Geometry check sheet. Reference: the model listing, model coordinates, mm. A direction names the side the tool comes from. Coordinates: 2 decimals unless noted, no trailing zeros. Write each loop counter-clockwise with the first axis right and the second up, starting at its lowest first coordinate (ties: lowest second). Pieces come first, ordered by that corner, then holes. Notation, with made-up numbers: (-19.75, 4.5) -> (0.25, 4.5) arc R12 cw to (0.25, 27.5) -> close; hole circle Ø2 at (-20, -6.75). An arc over 180 degrees is marked (long way). One line per question, with ' | ' between items.
Autodesk Inventor part; units mm, degrees
ref_plane "YZ Plane" through (0, 0, 0) normal (1, 0, 0) x (0, 1, 0)
ref_plane "XZ Plane" through (0, 0, 0) normal (0, 1, 0) x (-1, 0, 0)
ref_plane "XY Plane" through (0, 0, 0) normal (0, 0, 1) x (1, 0, 0)
sketch "Sketch1" plane through (0, 0, 0) normal (1, 0, 0) x (0, 1, 0)
  line L0 (0, 0) -> (16, 0)
  line L1 (16, 0) -> (16, -52)
  line L2 (16, -52) -> (0, -52)
  line L3 (0, -10) -> (0, -10)
  line L4 (0, -10) -> (0, -25)
  line L5 (0, -25) -> (0, -25)
  line L6 (0, -42) -> (0, -42)
  line L7 (0, -42) -> (0, -27)
  line L8 (0, -27) -> (0, -27)
  line L9 (0, -10) -> (0, 0)
  line L10 (0, -52) -> (0, -42)
  line L11 (0, -27) -> (0, -25)
  dimension "d0" = 16
  dimension "d1" = 52
  dimension "d2" = 0
  dimension "d3" = 15
  dimension "d4" = 10
  dimension "d5" = 15
  dimension "d6" = 10
  dimension "d10" = 0
  dimension "d11" = 0
  dimension "d12" = 0
extrude "Extrusion1" add sketch "Sketch1" along normal blind 2
sketch "Sketch3" plane through (2, 0, 0) normal (1, 0, 0) x (0, 0, -1)
  circle A0 centre (10, 8) radius 2.5
  circle A1 centre (32, 8) radius 2.5
  circle A2 centre (44, 8) radius 2.5
  line L0 (0, 16) -> (0, 0)
  line L1 (52, 16) -> (0, 16)
  dimension "d18" = 5
  dimension "d19" = 5
  dimension "d20" = 5
  dimension "d21" = 10
  dimension "d22" = 8
  dimension "d23" = 8
  dimension "d24" = 22
  dimension "d25" = 8
  dimension "d26" = 12
extrude "Extrusion3" cut sketch "Sketch3" against normal blind 10
sketch "Sketch4" plane through (0, 0, 0) normal (-1, 0, 0) x (0, 0, 1)
  circle A0 centre (-63.5, 35) radius 2.5
  circle A1 centre (-77, 8) radius 1.5
  circle A2 centre (-65, 8) radius 1.5
  line L0 (-58, -1) -> (-58, 17)
  line L1 (-84, 17) -> (-58, 17)
  line L2 (-84, 17) -> (-84, -1)
  line L3 (-58, -1) -> (-84, -1)
  line L4 (-51.8335, 14.6577) -> (-40.3589, 16)
  line L5 (-52, 16) -> (0, 16)
  line L6 (-72.4772, 16.1758) -> (-72.4069, 41.1757)
  line L7 (-72.4069, 41.1757) -> (-56.407, 41.1307)
  line L8 (-56.407, 41.1307) -> (-56.4773, 16.1308)
  line L9 (-51.8335, 14.6577) -> (-72.4308, 32.6757)
  line L10 (-72.4069, 41.1757) -> (-56.407, 41.1307)
  line L11 (-56.407, 41.1307) -> (-56.4381, 30.0657)
  line L12 (-40.3589, 16) -> (-56.4381, 30.0657)
  point P0 (0, 0)
extrude "Extrusion4" add sketch "Sketch4" against normal blind 2 contours L6 L7 L8 L9 | L8 L12 L4 L9
properties part number "Mounting_wall"
1. Cross-section at B-B on x = 1.35. Record the boundary of the cut face in (y, z), and give its area (3 significant figures).
Worked answers:
outline: (0, -52) -> (14.8, -52) -> (32.68, -72.43) -> (41.18, -72.41) -> (41.13, -56.41) -> (30.07, -56.44) -> (16, -40.36) -> (16, 0) -> (0, 0) -> close; hole circle Ø5 at (8, -44); hole circle Ø5 at (8, -32); hole circle Ø5 at (8, -10); hole circle Ø5 at (35, -63.5) | area: 1,110 mm²
2. Cross-section at A-A on z = -32. Record the boundary of the cut face in (x, y).
Worked answers:
outline: (0, 0) -> (2, 0) -> (2, 5.5) -> (0, 5.5) -> close; (0, 10.5) -> (2, 10.5) -> (2, 16) -> (0, 16) -> close
3. Go/stop test with flat-tipped pins: P1, Ø1, axis at y = 17.5, z = -32, coming from the -X side; P2, Ø1, axis at x = 0.5, y = 14, coming from the -Z side. Record where each tip stops, or that it passes through.
Worked answers:
P1: through | P2: z = -52
4. Material ranges on line 1 (Y direction, x = 0.6, z = -10); line 2 (Z direction, x = 0.3, y = 8.5); line 3 (Z direction, x = 0.4, y = 9), recorded low to high. Write a range as from..to.
Worked answers:
line 1: 0..5.5, 10.5..16 | line 2: -52..-46.45, -41.55..-34.45, -29.55..-12.45, -7.55..0 | line 3: -52..-46.29, -41.71..-34.29, -29.71..-12.29, -7.71..0
5. Cross-section at D-D on z = -44. Record the boundary of the cut face in (x, y).
Worked answers:
outline: (0, 0) -> (2, 0) -> (2, 5.5) -> (0, 5.5) -> close; (0, 10.5) -> (2, 10.5) -> (2, 19.19) -> (0, 19.19) -> close
6. Mould release check, pull along Z, two halves, no side actions. Record for faces 4 (the face through (1.01, 5.56, -9.46)), 5 (the face through (0, 15.7, -35.7)), 6 (the face through (1, 8, 0)), 7 (the face through (0.99, 23.61, -62.07)): released by +Z, released by -Z, zero draft, split by the parting line, or undercut.
Worked answers:
face 4: undercut | face 5: zero draft | face 6: released by +Z | face 7: released by -Z
7. Cross-section at C-C on y = 7. Record the boundary of the cut face in (x, z), and give its area (3 significant figures).
Worked answers:
outline: (0, -52) -> (2, -52) -> (2, -46.29) -> (0, -46.29) -> close; (0, -41.71) -> (2, -41.71) -> (2, -34.29) -> (0, -34.29) -> close; (0, -29.71) -> (2, -29.71) -> (2, -12.29) -> (0, -12.29) -> close; (0, -7.71) -> (2, -7.71) -> (2, 0) -> (0, 0) -> close | area: 76.5 mm²
8. Tool access check on faces 1 (the face through (0.99, 34.04, -61.19)), 2 (the face through (1, 16, -20)), 3 (the face through (1, 8, -52)). Record the directions out of +Z, -Z, +X, -X, +Y, -Y that give a thin tool (end or side, any length) a straight path to the whole face; none if there is none.
Worked answers:
face 1: +X, -X | face 2: +Z, +X, -X, +Y | face 3: -Z, +X, -X, -Y
